```python
from build123d import *

# Parameters (mm, degrees)
F0_W     = 80
F0_H     = 7.5
F0_R     = 2.25
F1_DEPTH = 2.5
F2_DEPTH = 5
F3_SIZE  = 1
F4_R     = 10
F5_R     = 5


with BuildPart() as f1:
    # F0 (on Top) → F1 (new body)
    with BuildSketch(Plane.XY):
        Rectangle(F0_W, F0_H)
        with BuildLine():
            Line((46.25, 10), (40, 3.75))
            Line((40, 3.75), (40, -3.75))
            Line((40, -3.75), (46.25, -10))
            Line((46.25, -10), (152.5, -10))
            ThreePointArc((152.5, -10), (162.5, 0), (152.5, 10))
            Line((152.5, 10), (46.25, 10))
        make_face()
        with Locations((152.5, 0)):
            Circle(F0_R, mode=Mode.SUBTRACT)
    extrude(amount=F1_DEPTH)

    # F0 (on Top) → F2 (join)
    with BuildSketch(Plane.XY):
        with BuildLine():
            Line((46.25, 10), (40, 3.75))
            Line((40, 3.75), (40, -3.75))
            Line((40, -3.75), (46.25, -10))
            Line((46.25, -10), (152.5, -10))
            ThreePointArc((152.5, -10), (162.5, 0), (152.5, 10))
            Line((152.5, 10), (46.25, 10))
        make_face()
        with Locations((152.5, 0)):
            Circle(F0_R, mode=Mode.SUBTRACT)
    extrude(amount=-F2_DEPTH)

    # F3
    f3_edges = [f1.edges().sort_by_distance(p)[0] for p in [
        (-40, -3.75, 1.25),
        (-40, 3.75, 1.25),
    ]]
    chamfer(f3_edges, length=F3_SIZE)

    # F4
    f4_edges = [f1.edges().sort_by_distance(p)[0] for p in [
        (40, -3.75, 1.25),
        (46.25, -10, -1.25),
        (46.25, 10, -1.25),
        (40, 3.75, 1.25),
    ]]
    fillet(f4_edges, radius=F4_R)

    # F5
    f5_edges = [f1.edges().sort_by_distance(p)[0] for p in [
        (40, -3.75, -2.5),
        (40, 3.75, -2.5),
    ]]
    fillet(f5_edges, radius=F5_R)


solid = f1.part
```
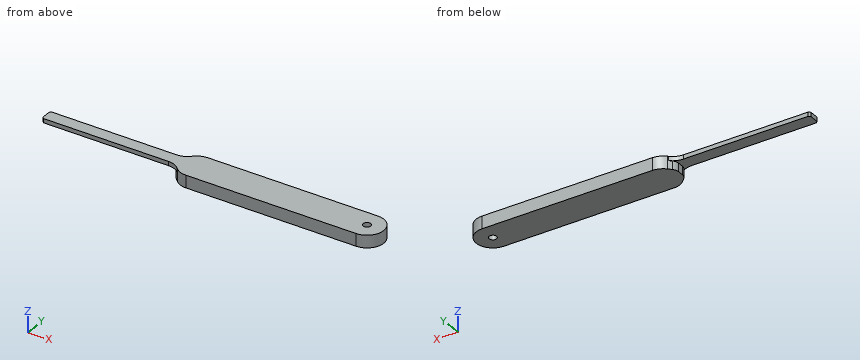
Read the model definition and answer for the solid it produces. Units are mm, in the model's axes. Coordinates: 2 decimals unless noted, no trailing zeros. Write each loop counter-clockwise with the first axis right and the second up, starting at its lowest first coordinate (ties: lowest second). Pieces come first, ordered by that corner, then holes. Notation, with made-up numbers: (65, 82.25) -> (103, 82.25) arc R16 cw to (103, 100.25) -> close; hole circle Ø2 at (21, -37.5). An arc over 180 degrees is marked (long way). Answer as a JSON object with one key per item and string values.
Q1. The part is cut by section C-C on x = -27. Give the vertices of the cut face in (y, z), then the cut area to 4 significant figures.
The answers:
{"outline": "(-3.75, 0) -> (3.75, 0) -> (3.75, 2.5) -> (-3.75, 2.5) -> close", "area": "18.75 mm2"}
Q2. The part is cut by section B-B on y = 0. Give the vertices of the cut face in (x, z), then the cut area to 4 significant figures.
The answers:
{"outline": "(-40, 0) -> (40, 0) -> (40, -5) -> (150.25, -5) -> (150.25, 2.5) -> (-40, 2.5) -> close; (154.75, -5) -> (162.5, -5) -> (162.5, 2.5) -> (154.75, 2.5) -> close", "area": "1,085 mm2"}
Q3. The part is cut by section A-A on z = -2. Give the vertices of the cut face in (x, y).
The answers:
{"outline": "(40, -1.68) arc R5 ccw to (41.46, -5.21) -> (43.32, -7.07) arc R10 ccw to (50.39, -10) -> (152.5, -10) arc R10 ccw to (152.5, 10) -> (50.39, 10) arc R10 ccw to (43.32, 7.07) -> (41.46, 5.21) arc R5 ccw to (40, 1.68) -> close; hole circle Ø4.5 at (152.5, 0)"}
Q4. Flat-ended cylindrical pins translate along their axes: pin 1 Ø10.5 at (x, y) = (8.5, 1) entering from -Z; pin 2 Ø1.7 at (y, z) = (-0.5, -2) entering from -X; pin 3 Ø2 at (x, z) = (9.5, 1) entering from -Y; pin 4 Ø1.5 at (x, y) = (-19.5, -6) entering from +Z. Find the tip coordinate at first contact, or state that the pin passes through.
The answers:
{"pin 1": "stops at z = 0", "pin 2": "stops at x = 40", "pin 3": "stops at y = -3.75", "pin 4": "passes through"}
Q5. Consider line 1 (X direction, y = 0.25, z = 1); line 2 (Y direction, x = 152.5, z = -1.25); line 3 (Z direction, x = -14, y = -2). Determine where each line is inside the solid, lowest interval first. Write a range as [from, to].
The answers:
{"line 1": "x = [-40, 150.26], [154.74, 162.5]", "line 2": "y = [-10, -2.25], [2.25, 10]", "line 3": "z = [0, 2.5]"}
